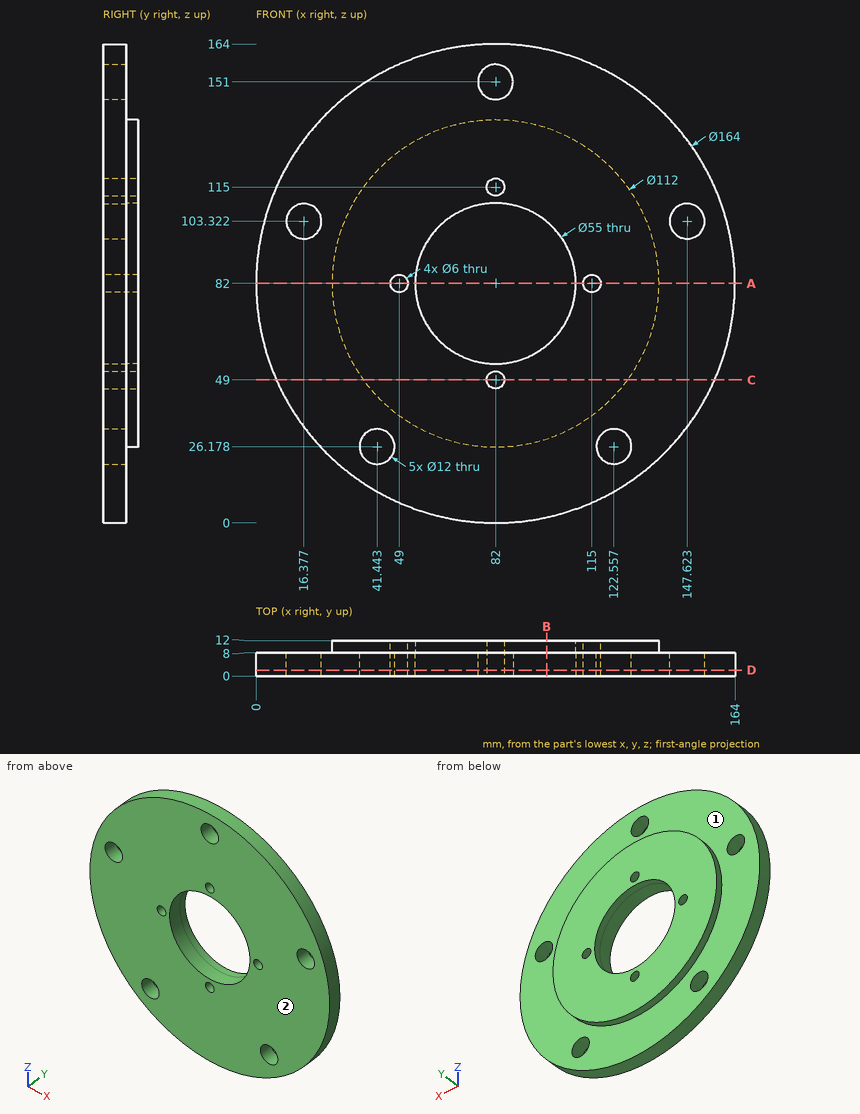
Study the drawing (mm; zero at the part's minimum x, y, z) and answer. A direction names the side the tool comes from. Give positions to 0.01 mm unless a question says otherwise; leave off trailing zeros. Order: outer loops, then holes, each group sorted by start corner. A loop starts at its lowest first (then second) coordinate and runs counter-clockwise, first axis right, second up. Notation, with made-up numbers: (-11, 45) - (4, 45) arc R15 ccw to (4, 59) - close; hole circle Ø3 at (89, -18). An arc over 180 degrees is marked (long way). Use one line per item in the form item = value. Start each with the question number.
(1) A cutting plane is placed at D-D, the plane y = 2. State how many separate pieces and enclosed holes the cut face has, then the cut area to 3 significant figures.
(2) For the marked faces 1 and 2, determine the directions among +Z, -Z, +X, -X, +Y, -Y from which every point of the face is accessible in a straight line to the end or side of a thin tool.
(3) A cutting plane is placed at A-A, the plane z = 82. Write down the section's boundary in (x, y).
(4) Flat-ended cylindrical pins translate along their axes: pin 1 Ø9.5 at (x, z) = (82, 151) entering from +Y; pin 2 Ø6 at (x, y) = (90.5, 2) entering from -Z; pin 3 Ø1.5 at (y, z) = (4.5, 137.5) entering from -X (1 decimal); pin 4 Ø3 at (x, z) = (96, 20.5) entering from +Y. Find the tip coordinate at first contact, or state that the pin passes through.
(5) A cutting plane is placed at B-B, the plane x = 99.5. Write down the section's boundary in (y, z).
(6) Consider line 1 (Z direction, x = 82, y = 5.25); line 2 (X direction, y = 1.5, z = 80) (1 decimal); line 3 (X direction, y = 6.5, z = 29.5). Determine where each line is inside the solid, lowest interval first. Write a range as from..to.
(7) A cutting plane is placed at C-C, the plane z = 49. Write down the section's boundary in (x, y).
Ans:
q1.separate_pieces = 1
q1.enclosed_holes = 10
q1.area = 18,100 mm^2
q2.face_1 = +Y
q2.face_2 = +Z, -Z, +X, -X, -Y
q3.outline = (0, 0) - (46, 0) - (46, 12) - (26, 12) - (26, 8) - (0, 8) - close; (52, 0) - (54.5, 0) - (54.5, 12) - (52, 12) - close; (109.5, 0) - (112, 0) - (112, 12) - (109.5, 12) - close; (118, 0) - (164, 0) - (164, 8) - (138, 8) - (138, 12) - (118, 12) - close
q4.pin_1 = through
q4.pin_2 = 0.18
q4.pin_3 = 21
q4.pin_4 = 8
q5.outline = (0, 1.89) - (8, 1.89) - (8, 28.8) - (12, 28.8) - (12, 60.79) - (0, 60.79) - close; (0, 103.21) - (12, 103.21) - (12, 135.2) - (8, 135.2) - (8, 162.11) - (0, 162.11) - close
q6.line_1 = 0..46, 52..54.5, 109.5..112, 118..145, 157..164
q6.line_2 = 0..46.8, 51.2..54.6, 109.4..112.8, 117.2..164
q6.line_3 = 19.01..36.45, 46.44..117.56, 127.55..144.99
q7.outline = (6.93, 0) - (79, 0) - (79, 12) - (36.76, 12) - (36.76, 8) - (6.93, 8) - close; (85, 0) - (157.07, 0) - (157.07, 8) - (127.24, 8) - (127.24, 12) - (85, 12) - close
